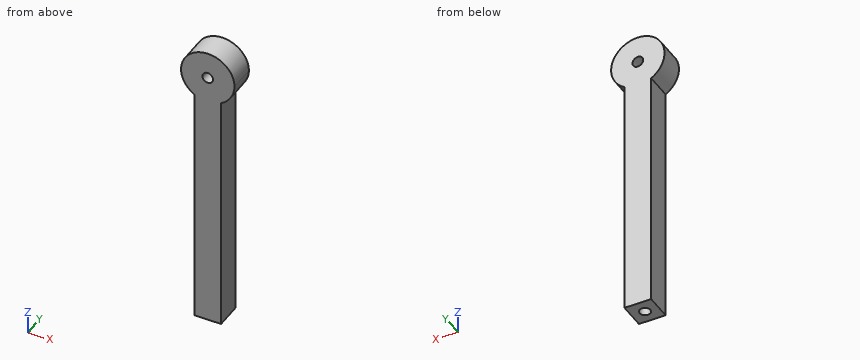
```python
from build123d import *

# Parameters (mm, degrees)
F1_DEPTH = 25
F2_DEPTH = 25
F4_D     = 10
F4_DEPTH = 140
F4_TIP   = 3.0043030951
F6_D     = 10


with BuildPart() as f1:
    # F0 (on Front) → F1 (new body)
    with BuildSketch(Plane.XZ):
        with BuildLine():
            Line((-12.5, 103.3493649054), (-12.5, -125))
            Line((-12.5, -125), (12.5, -125))
            Line((12.5, -125), (12.5, 103.3493649054))
            ThreePointArc((12.5, 103.3493649054), (0, 100), (-12.5, 103.3493649054))
        make_face()
    extrude(amount=F1_DEPTH)

    # F0 (on Front) → F2 (join)
    with BuildSketch(Plane.XZ):
        with BuildLine():
            Line((-12.5, 103.3493649054), (-12.5, -125))
            Line((-12.5, -125), (12.5, -125))
            Line((12.5, -125), (12.5, 103.3493649054))
            ThreePointArc((12.5, 103.3493649054), (0, 100), (-12.5, 103.3493649054))
        make_face()
        with BuildLine():
            ThreePointArc((25, 125), (-12.5, 146.6506350946), (-12.5, 103.3493649054))
            Line((-12.5, 103.3493649054), (-12.5, 125))
            Line((-12.5, 125), (12.5, 125))
            Line((12.5, 125), (12.5, 103.3493649054))
            ThreePointArc((12.5, 103.3493649054), (21.6506350946, 112.5), (25, 125))
        make_face()
        with BuildLine():
            Line((-12.5, 125), (-12.5, 103.3493649054))
            ThreePointArc((-12.5, 103.3493649054), (0, 100), (12.5, 103.3493649054))
            Line((12.5, 103.3493649054), (12.5, 125))
            Line((12.5, 125), (-12.5, 125))
        make_face()
    extrude(amount=F2_DEPTH)

    # F4
    with Locations(Plane(origin=(0, 0, -125), x_dir=(1, 0, 0), z_dir=(0, 0, -1))):
        with Locations((0, 12.5)):
            Hole(F4_D / 2, depth=F4_DEPTH)
            with Locations((0, 0, -(F4_DEPTH + F4_TIP / 2))):  # 118° drill point
                Cone(0, F4_D / 2, F4_TIP, mode=Mode.SUBTRACT)

    # F6 (through all)
    with Locations(Plane.XZ.offset(25)):
        with Locations((0, 125)):
            Hole(F6_D / 2)


solid = f1.part
```
Input: part model. Units: mm. Frame: model coordinates. Give positions to 0.01 mm unless a question says otherwise; leave off trailing zeros. Order: outer loops, then holes, each group sorted by start corner. A loop starts at its lowest first (then second) coordinate and runs counter-clockwise, first axis right, second up. Notation, with made-up numbers: (53, 81) -> (75, 81) arc R21 cw to (75, 101) -> close; hole circle Ø10 at (75, 80.25). An arc over 180 degrees is marked (long way). Write each question's results on one line, items separated by ' | '. Start each with the question number.
Item 1: Cut plane C-C on x = -18. Return the cut outline in (y, z), then the cut area to 3 significant figures.
Item 2: Cut plane B-B on y = -22.75. Return the cut outline in (x, z).
Item 3: Cut plane A-A on z = -68.5. Return the cut outline in (x, y).
Item 4: Line query: line 1 (Y direction, x = 0, z = -67.5); line 2 (Z direction, x = 0, y = -6); line 3 (X direction, y = -12, z = -77.5). Output: solid intervals per line, ascending.
Item 5: Contact query for flat-ended pins moving along their axis: P1, Ø2, axis at x = -4.5, y = -22, coming from the +Z side; P2, Ø1.5, axis at y = -10.5, z = 96.5, coming from the +X side; P3, Ø12, axis at x = 18, y = -8, coming from the +Z side. Output: stop coordinate, or through.
Item 6: Cut plane D-D on z = 40. Return the cut outline in (x, y), then the cut area to 3 significant figures.
Established:
1) outline: (-25, 107.65) -> (0, 107.65) -> (0, 142.35) -> (-25, 142.35) -> close | area: 867 mm^2
2) outline: (-12.5, -125) -> (12.5, -125) -> (12.5, 103.35) arc R25 ccw (long way) to (-12.5, 103.35) -> close; hole circle Ø10 at (0, 125)
3) outline: (-12.5, -25) -> (12.5, -25) -> (12.5, 0) -> (-12.5, 0) -> close; hole circle Ø10 at (0, -12.5)
4) line 1: -25 to -17.5, -7.5 to 0 | line 2: -125 to 120, 130 to 150 | line 3: -12.5 to -4.97, 4.97 to 12.5
5) P1: z = 149.75 | P2: x = 12.5 | P3: z = 146.93
6) outline: (-12.5, -25) -> (12.5, -25) -> (12.5, 0) -> (-12.5, 0) -> close | area: 625 mm^2
